```python
from build123d import *

# Parameters (mm, degrees)
F0_W     = 70
F0_H     = 40
F1_DEPTH = 12.5
F2_T     = -2.5
F4_R     = 5.76607
F4_R_2   = 5.765
F5_DEPTH = 65


with BuildPart() as f1:
    # F0 (on Top) → F1 (new body)
    with BuildSketch(Plane.XY):
        Rectangle(F0_W, F0_H)
    extrude(amount=F1_DEPTH)

    # F2
    f2_openings = [f1.faces().sort_by_distance(p)[0] for p in [
        (0, 0, 12.5),
    ]]
    offset(amount=F2_T, openings=f2_openings)

    # F4 (on offset) → F5 (join)
    with BuildSketch(Plane.YZ.offset(-32.5)):
        with Locations((0, 6.708693)):
            Circle(F4_R)
        with Locations((12.160433, 6.742671)):
            Circle(F4_R_2)
        with Locations((-12.139365, 6.572861)):
            Circle(F4_R_2)
    extrude(amount=F5_DEPTH)


solid = f1.part
```
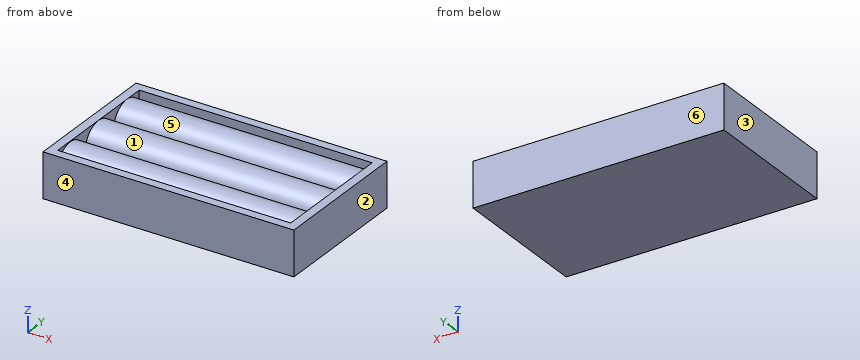
Could you check a few things on this model? Use its own coordinates, in mm. Face numbers are marked on the shaded views. A direction names the side the tool comes from. Round coordinates to 2 decimals unless told otherwise and drop trailing zeros. Loops run counter-clockwise (first coordinate to the right, second up) from the corner with the lowest first, then second, coordinate; pieces in that order, holes last.
Q1. I want a section at B-B (z = 6.25). Write out the boundary of the cut face in (x, y), and give its area (3 significant figures).
Q2. I want a section at A-A (x = 18). Write out the boundary of the cut face in (y, z) (3 decimals).
Q3. For P1, Ø2, axis at x = -12.5, y = 5.5, coming from the +Z side; P2, Ø8, axis at x = -24.5, y = -7, coming from the +Z side; P3, Ø0.6, axis at x = 13, y = -17, coming from the +Z side, each with a flat end and sliding along its axis, tell me the tip position at first contact or that it passes through.
Q4. Please list where these lines run through material, in increasing order: L1, parallel to Y at x = -30, z = 7; L2, parallel to Y at x = -0.5, z = 3 (1 decimal); L3, parallel to Y at x = -17.5, z = 7.5.
Q5. On a 3-axis mill with a long thin cutter (end or side, diameter ignored), from which of +Z, -Z, +X, -X, +Y, -Y can I reach the whole of each face in a straight line? I mean the marked faces 5 and 6. Say none if no direction works.
Q6. Thinking about a two-plate mould opening in X: for the marked faces 1, 2, 3 and 4, which applies, pulls with the +X half, pulls with the -X half, needs draft (parallel to the pull), parting line crosses it, or undercut?
Q7. I want a section at D-D (y = 15). Write out the boundary of the cut face in (x, z), and give its area (3 significant figures).
Q8. I want a section at C-C (y = -2). Write out the boundary of the cut face in (x, z), and give its area (3 significant figures).
Answer below:
1. outline: (-35, -20) - (35, -20) - (35, 20) - (-35, 20) - close; hole (-32.5, -6.38) - (32.5, -6.38) - (32.5, -5.75) - (-32.5, -5.75) - close; hole (-32.5, 5.75) - (32.5, 5.75) - (32.5, 6.42) - (-32.5, 6.42) - close
1. area: 2,720 mm2
2. outline: (-20, 0) - (20, 0) - (20, 12.5) - (17.5, 12.5) - (17.5, 8.916) arc R5.765 ccw (long way) to (8.257, 2.5) - (3.941, 2.5) arc R5.766 ccw (long way) to (-3.941, 2.5) - (-8.059, 2.5) arc R5.765 ccw (long way) to (-17.5, 8.694) - (-17.5, 12.5) - (-20, 12.5) - close; hole (-17.5, 2.5) - (-16.219, 2.5) arc R5.765 cw to (-17.5, 4.452) - close; hole (16.064, 2.5) - (17.5, 2.5) - (17.5, 4.569) arc R5.765 cw to start
3. P1: stops at z = 10.31
3. P2: stops at z = 12.22
3. P3: stops at z = 10.1
4. L1: y = -20 to -6.39, -5.76 to 5.76, 6.4 to 20
4. L2: y = -20 to -17.5, -16.7 to -7.6, -4.4 to 4.4, 7.8 to 16.5, 17.5 to 20
4. L3: y = -20 to -6.45, -5.71 to 5.71, 6.45 to 20
5. face 5: none
5. face 6: +Z, -Z, +X, -X, +Y
6. face 1: undercut
6. face 2: pulls with the +X half
6. face 3: pulls with the -X half
6. face 4: needs draft
7. outline: (-35, 0) - (35, 0) - (35, 12.5) - (32.5, 12.5) - (32.5, 11.76) - (-32.5, 11.76) - (-32.5, 12.5) - (-35, 12.5) - close
7. area: 827 mm2
8. outline: (-35, 0) - (35, 0) - (35, 12.5) - (32.5, 12.5) - (32.5, 12.12) - (-32.5, 12.12) - (-32.5, 12.5) - (-35, 12.5) - close
8. area: 850 mm2
